Read the model definition and answer for the solid it produces. Units are mm, in the model's axes. A direction names the side the tool comes from. Coordinates: 2 decimals unless noted, no trailing zeros. Order: outer loops, then holes, each group sorted by start corner. A loop starts at its lowest first (then second) coordinate and runs counter-clockwise, first axis right, second up. Notation, with made-up numbers: (88.5, 38) - (139.5, 38) arc R26 cw to (139.5, 52) - close; hole circle Ø8 at (54, 53). An arc over 180 degrees is marked (long way). Write item = value, one per line.
from build123d import *

# Parameters (mm, degrees)
F0_W      = 21
F0_H      = 14
F1_DEPTH  = 3
F2_W      = 7
F2_H      = 14
F3_DEPTH  = 1.5
F5_W      = 80
F5_H      = 50
F6_DEPTH  = 2
F8_DEPTH  = 1
F10_DEPTH = 2


with BuildPart() as f1:
    # F0 (on Top) → F1 (new body)
    with BuildSketch(Plane.XY):
        Rectangle(F0_W, F0_H)
    extrude(amount=F1_DEPTH)

    # F2 (on face) → F3 (join)
    with BuildSketch(Plane.XY.offset(3)):
        Rectangle(F2_W, F2_H)
    extrude(amount=F3_DEPTH)

    # F4: F1 across face


with BuildPart() as f1_1:
    add(f1.part)
    add(f1.part.mirror(Plane.XY.offset(4.5)))

    # F5 (on face) → F6 (join)
    with BuildSketch(Plane.XY.offset(9)):
        with Locations((0, -18)):
            Rectangle(F5_W, F5_H)
    extrude(amount=F6_DEPTH)

    # F7 (on face) → F8 (join)
    with BuildSketch(Plane.XY.offset(11)):
        Polygon((-38, 7), (-40, 7), (-40, -43), (40, -43), (40, 7), (38, 7), (38, -41), (-38, -41), align=None)
    extrude(amount=F8_DEPTH)

    # F9 (on face) → F10 (join)
    with BuildSketch(Plane.XY.offset(12)):
        Polygon((-35, 7), (-40, 7), (-40, -43), (40, -43), (40, 7), (35, 7), (35, -38), (-35, -38), align=None)
    extrude(amount=F10_DEPTH)


solid = f1_1.part
1) Flat-ended cylindrical pins translate along their axes: pin 1 Ø2.5 at (y, z) = (1.5, 4.5) entering from +X; pin 2 Ø1 at (x, z) = (-9, 13) entering from +Y; pin 3 Ø5.5 at (x, y) = (-7.5, 0) entering from +Z; pin 4 Ø2 at (x, y) = (5.5, 3.5) entering from -Z. Find the tip coordinate at first contact, or state that the pin passes through.
Returned:
pin_1 = 3.5
pin_2 = -38
pin_3 = 11
pin_4 = 0
2) Straight lines are drawn through the part: line 1 along X through (y, z) = (2.5, 13.5); line 2 along Z through (x, y) = (18, -2); line 3 along Z through (x, y) = (-26.5, -39). For each, find the intervals that lie inside material, in ascending order. Write a range as from..to.
Returned:
line_1 = -40..-35, 35..40
line_2 = 9..11
line_3 = 9..11, 12..14
3) Determine the mould class of faces 6 (the face through (2.8, -38.3, 14)), 7 (the face through (-7, 0, 3)), 8 (the face through (-10.5, 0, 8)) for opening direction Z: pulls with the +Z half, pulls with the -Z half, needs draft (parallel to the pull), parting line crosses it, or undercut.
Returned:
face_6 = pulls with the +Z half
face_7 = undercut
face_8 = needs draft
4) For faces 1 (the face through (0, -7, 5)), 2 (the face through (-0.2, -38.2, 12)), 3 (the face through (-3.5, 0, 5)), 4 (the face through (-10.5, 0, 1)), 5 (the face through (10.5, 0, 1)), determine the directions among +Z, -Z, +X, -X, +Y, -Y from which every point of the face is accessible in a straight line to the end or side of a thin tool.
Returned:
face_1 = -Z, +X, -X, -Y
face_2 = +Y
face_3 = -X, +Y, -Y
face_4 = -Z, -X, +Y, -Y
face_5 = -Z, +X, +Y, -Y
5) The part is cut by section C-C (x = -20.5). Determine the outline of the cut face in (y, z).
Returned:
outline = (-43, 9) - (7, 9) - (7, 11) - (-41, 11) - (-41, 12) - (-38, 12) - (-38, 14) - (-43, 14) - close
6) The part is cut by section A-A (x = -7). Determine the outline of the cut face in (y, z).
Returned:
outline = (-43, 9) - (-7, 9) - (-7, 6) - (7, 6) - (7, 11) - (-41, 11) - (-41, 12) - (-38, 12) - (-38, 14) - (-43, 14) - close; (-7, 0) - (7, 0) - (7, 3) - (-7, 3) - close
7) The part is cut by section B-B (y = -23). Determine the outline of the cut face in (x, z).
Returned:
outline = (-40, 9) - (40, 9) - (40, 14) - (35, 14) - (35, 12) - (38, 12) - (38, 11) - (-38, 11) - (-38, 12) - (-35, 12) - (-35, 14) - (-40, 14) - close
8) The part is cut by section D-D (z = 1.5). Determine the outline of the cut face in (x, y), and give its area (3 significant figures).
Returned:
outline = (-10.5, -7) - (10.5, -7) - (10.5, 7) - (-10.5, 7) - close
area = 294 mm^2
